Autodesk Inventor part; units mm, degrees
ref_plane "Arbeitsebene1" through (0, 0, 3) normal (0, 0, 1) x (1, 0, 0)
ref_plane "YZ Plane" through (0, 0, 0) normal (1, 0, 0) x (0, 1, 0)
ref_plane "XZ Plane" through (0, 0, 0) normal (0, 1, 0) x (-1, 0, 0)
sketch "Skizze1" plane through (0, 0, 0) normal (0, 0, 1) x (1, 0, 0)
  circle A0 centre (0, 0) radius 60
  dimension "d0" = 120
extrude "Extrusion1" add sketch "Skizze1" along normal blind 6
ref_plane "Arbeitsebene1" through (0, 0, 3) normal (0, 0, 1) x (1, 0, 0)
sketch "Skizze3" plane through (0, 0, 3) normal (0, 0, 1) x (1, 0, 0)
  circle A0 centre (0, 0) radius 25
  dimension "d5" = 50
extrude "Extrusion2" add sketch "Skizze3" along normal mid plane 12
sketch "Skizze4" plane through (0, 0, 9) normal (0, 0, 1) x (1, 0, 0)
  circle A0 centre (0, 0) radius 22.5
  dimension "d8" = 45
extrude "Extrusion3" cut sketch "Skizze4" against normal blind 12
fillet "Rundung1" radius 2 1 edges at (-25, 0, 6)
fillet "Rundung2" radius 2 1 edges at (-25, 0, 0)
sketch "Skizze5" plane through (0, 0, 6) normal (0, 0, 1) x (1, 0, 0)
  line L0 (25.4807, -45) -> (-25.4807, -45)
  arc A0 (-20.3044, -25.6815) -> (20.3044, -25.6815) centre (0, 0) ccw
  circle A1 centre (0, 0) radius 27
  line L1 (20.3044, -25.6815) -> (25.4807, -45)
  line L2 (-20.3044, -25.6815) -> (-25.4807, -45)
  line L3 (0, 0) -> (0, -59.7048) construction
  circle A2 centre (0, 0) radius 22.5
  dimension "d16" = 20
  dimension "d17" = 45
  dimension "d18" = 75
extrude "Extrusion4" cut sketch "Skizze5" against normal blind 12 contours L0 L2 A0 L1
fillet "Rundung3" radius 2 2 edges at (-25.4807, -45, 3) (25.4807, -45, 3)
fillet "Rundung4" radius 2 2 edges at (-20.3044, -25.6815, 3) (20.3044, -25.6815, 3)
pattern_circular "Runde Anordnung1" count 4 over 360 about axis through (0, 0, 0) along (0, 0, 1) of "Extrusion4", "Rundung4", "Rundung3"
fillet "Rundung5" radius 1 2 edges at (-60, 0, 0) (-60, 0, 6)
properties part number "practice6" material "Stahl, galvanisiert"
Here's how the part is built. I have some questions about the finished solid (model axes, mm). A direction names the side the tool comes from. Coordinates: 2 decimals unless noted, no trailing zeros.
1. I need wall thicknesses on L1, parallel to Y at x = 0, z = 1.25; L2, parallel to Y at x = -13.5, z = 4.5; L3, parallel to X at y = -16, z = 3.5. Which ranges of each line are inside material? Lowest first, please.
2. For faces 4 (the cylindrical face through (0.267, 32.737, 3.042)), 5 (the cylindrical face through (23.846, -7.509, 8.493)), which set-ups out of +Z, -Z, +X, -X, +Y, -Y let a thin tool reach every point of the face, with its end or its side?
3. If we mould it in two halves opening along X, with no side actions, what happens to faces 1 (the cylindrical face through (-59.94, -2.64, 2.97)), 2 (the flat face through (-22.34, 3.82, -3)), 3 (the cylindrical face through (32.737, -0.267, 3.042))? For each: pulls with the +X half, pulls with the -X half, needs draft (parallel to the pull), parting line crosses it, or undercut.
4. Imagine slicing it at A-A, the plane x = 0. Count the separate pieces of the cut face and the enclosed holes in it, and give its area (3 significant figures).
5. For P1, Ø5, axis at y = -3, z = 4, coming from the +X side; P2, Ø1.8, axis at y = -0.5, z = 3, coming from the -X side; P3, Ø4, axis at y = -38, z = 4, coming from the +X side; P4, Ø4, axis at y = 31, z = 7.5, coming from the +X side, each with a flat end and sliding along its axis, tell me the tip position at first contact or that it passes through.
Taken from the geometry:
1. L1: y = -60 to -45, -32.74 to -22.5, 22.5 to 32.74, 45 to 60
1. L2: y = -58.46 to -45, -29.83 to -18, 18 to 29.83, 45 to 58.46
1. L3: x = -57.83 to -45, -28.56 to -15.82, 15.82 to 28.56, 45 to 57.83
2. face 4: +Z, -Z
2. face 5: +Z
3. face 1: parting line crosses it
3. face 2: needs draft
3. face 3: undercut
4. separate pieces: 4
4. enclosed holes: 0
4. area: 335 mm2
5. P1: stops at x = 60
5. P2: stops at x = -60
5. P3: stops at x = 48
5. P4: stops at x = 51.56
